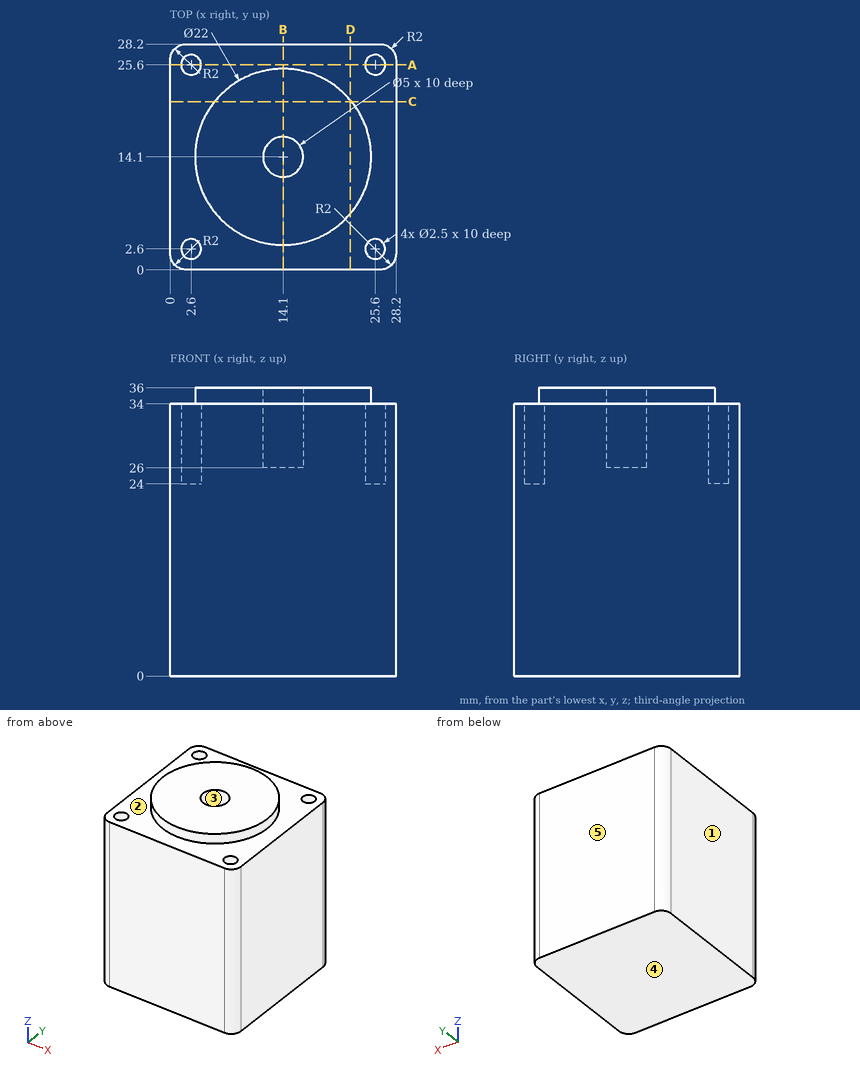
Input: dimensioned drawing with shaded views. Units: mm. Origin: part minimum x, y, z. A direction names the side the tool comes from. Give positions to 0.01 mm unless a question says otherwise; leave off trailing zeros. Write each loop counter-clockwise with the first axis right and the second up, starting at its lowest first coordinate (ties: lowest second). Pieces come first, ordered by that corner, then holes.
1. Section query C-C, the plane y = 21. Return loops of the section in (x, z).
2. Section query B-B, the plane x = 14.1. Return loops of the section in (y, z), then the cut area to 3 significant figures.
3. Section query A-A, the plane y = 25.6. Return loops of the section in (x, z), then the cut area to 3 significant figures.
4. Reachability of the marked faces 1 and 2 from +Z, -Z, +X, -X, +Y, -Y: full face, straight path, thin tool, end or side. Return the list, or none.
5. Line query: probe 1 along Y at (x, z) = (2.6, 29.5); probe 2 along Y at (x, z) = (3.25, 29.5). Output: solid intervals per line, ascending.
6. Draft query along Y for the marked faces 3, 4 and 5. Return one class per face: released by +Y, released by -Y, zero draft, split by the parting line, or undercut.
7. Section query D-D, the plane x = 22.5. Return loops of the section in (y, z).
8. Pin query (flat end, axial travel): P1, Ø6, axis at y = 5, z = 19.5, coming from the -X side; P2, Ø1.5, axis at x = 2.6, y = 2.6, coming from the +Z side; P3, Ø3, axis at x = 25.5, y = 2, coming from the +Z side; P4, Ø1.5, axis at x = 14.5, y = 14.5, coming from the +Z side. Return the tip coordinate at first contact, or that it passes through.
Computed:
1. outline: (0, 0) - (28.2, 0) - (28.2, 34) - (22.67, 34) - (22.67, 36) - (5.53, 36) - (5.53, 34) - (0, 34) - close
2. outline: (0, 0) - (28.2, 0) - (28.2, 34) - (25.1, 34) - (25.1, 36) - (16.6, 36) - (16.6, 26) - (11.6, 26) - (11.6, 36) - (3.1, 36) - (3.1, 34) - (0, 34) - close
2. area: 953 mm2
3. outline: (0, 0) - (28.2, 0) - (28.2, 34) - (26.85, 34) - (26.85, 24) - (24.35, 24) - (24.35, 34) - (3.85, 34) - (3.85, 24) - (1.35, 24) - (1.35, 34) - (0, 34) - close
3. area: 909 mm2
4. face 1: +Z, -Z, -X, +Y, -Y
4. face 2: +Z
5. probe 1: y = 0 to 1.35, 3.85 to 24.35, 26.85 to 28.2
5. probe 2: y = 0 to 1.53, 3.67 to 24.53, 26.67 to 28.2
6. face 3: undercut
6. face 4: zero draft
6. face 5: released by +Y
7. outline: (0, 0) - (28.2, 0) - (28.2, 34) - (21.2, 34) - (21.2, 36) - (7, 36) - (7, 34) - (0, 34) - close
8. P1: stops at x = 0
8. P2: stops at z = 24
8. P3: stops at z = 34
8. P4: stops at z = 26
